from build123d import *

# Parameters (mm, degrees)
SKETCH1_W               = 50.8
SKETCH1_H               = 36.83
BOSS_EXTRUDE1_DEPTH     = 8.89
SKETCH2_W               = 36.83
SKETCH2_H               = 8.89
BOSS_EXTRUDE2_DEPTH     = 0.254
SKETCH3_W               = 4.318
SKETCH3_H               = 10.16
BOSS_EXTRUDE3_DEPTH     = 20.32
CUT_EXTRUDE1_DEPTH      = 54.86357322
CUT_EXTRUDE1_DEPTH_BACK = 54.86357322
SKETCH4_R               = 2.54
FILLET1_R               = 3.81
SKETCH18_5_W            = 20.32
SKETCH18_5_H            = 2.54
CUT_EXTRUDE2_DEPTH      = 51.556369539
SKETCH7_W               = 20.32
SKETCH7_H               = 2.54
CUT_EXTRUDE3_DEPTH      = 51.556369539
SKETCH18_16_R           = 1.27
BOSS_EXTRUDE4_DEPTH     = 6.35
FILLET2_R               = 2.032


with BuildPart() as part:
    # Sketch1 → Boss-Extrude1 (new body)
    with BuildSketch(Plane(origin=(0, 0, 0), x_dir=(1, 0, 0), z_dir=(0, 1, 0))):
        Rectangle(SKETCH1_W, SKETCH1_H)
    extrude(amount=-BOSS_EXTRUDE1_DEPTH)

    # Sketch2 → Boss-Extrude2 (add)
    with BuildSketch(Plane(origin=(25.4, 0, 0), x_dir=(0, 0, -1), z_dir=(1, 0, 0))):
        with Locations((0, -4.445)):
            Rectangle(SKETCH2_W, SKETCH2_H)
    extrude(amount=BOSS_EXTRUDE2_DEPTH)

    # Sketch3 → Boss-Extrude3 (add)
    with BuildSketch(Plane(origin=(25.654, 0, 0), x_dir=(0, 0, -1), z_dir=(1, 0, 0))):
        with Locations((-5.588, -5.08)):
            Rectangle(SKETCH3_W, SKETCH3_H)
        with Locations((5.588, -5.08)):
            Rectangle(SKETCH3_W, SKETCH3_H)
    extrude(amount=BOSS_EXTRUDE3_DEPTH)

    # Sketch4 → Cut-Extrude1 (cut, two sides: drawn at the far end of the back side and taken through both)
    with BuildSketch(Plane(origin=(0, 0, -7.747), x_dir=(-1, 0, 0), z_dir=(0, 0, -1)).offset(-CUT_EXTRUDE1_DEPTH_BACK)):
        with Locations((-40.894, -4.445)):
            Circle(SKETCH4_R)
    extrude(amount=CUT_EXTRUDE1_DEPTH + CUT_EXTRUDE1_DEPTH_BACK, mode=Mode.SUBTRACT)

    # Fillet1
    fillet1_edges = [part.edges().sort_by_distance(p)[0] for p in [
        (45.974, 0, 5.588),
        (45.974, -10.16, 5.588),
        (45.974, 0, -5.588),
        (45.974, -10.16, -5.588),
    ]]
    fillet(fillet1_edges, radius=FILLET1_R)

    # Sketch18_5 → Cut-Extrude2 (cut, through all)
    with BuildSketch(Plane(origin=(0, 0, 0), x_dir=(1, 0, 0), z_dir=(0, 1, 0))):
        with Locations((12.7, 16.256)):
            Rectangle(SKETCH18_5_W, SKETCH18_5_H)
    extrude(amount=-CUT_EXTRUDE2_DEPTH, mode=Mode.SUBTRACT)

    # Sketch7 → Cut-Extrude3 (cut, through all)
    with BuildSketch(Plane(origin=(0, 0, 0), x_dir=(1, 0, 0), z_dir=(0, 1, 0))):
        with Locations((12.7, -16.256)):
            Rectangle(SKETCH7_W, SKETCH7_H)
    extrude(amount=-CUT_EXTRUDE3_DEPTH, mode=Mode.SUBTRACT)

    # Sketch18_16 → Boss-Extrude4 (add)
    with BuildSketch(Plane(origin=(0, 0, 0), x_dir=(1, 0, 0), z_dir=(0, 1, 0))):
        with Locations(Location((-19.304, -14.732, 0), (0, 0, 270))):
            Circle(SKETCH18_16_R)
        with Locations(Location((-19.304, 14.732, 0), (0, 0, 270))):
            Circle(SKETCH18_16_R)
    extrude(amount=BOSS_EXTRUDE4_DEPTH)

    # Fillet2
    fillet2_edges = [part.edges().sort_by_distance(p)[0] for p in [
        (-19.304, 0, 13.462),
        (-19.304, 0, -16.002),
    ]]
    fillet(fillet2_edges, radius=FILLET2_R)


solid = part.part
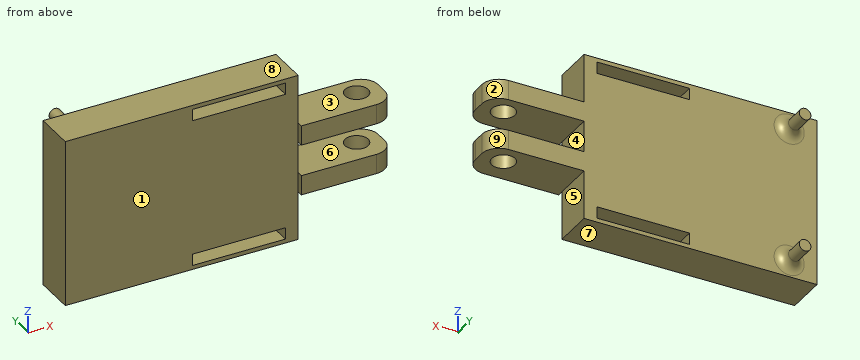
Could you check a few things on this model? Use its own coordinates, in mm. Face numbers are marked on the shaded views. A direction names the side the tool comes from. Give positions to 0.01 mm unless a question says otherwise; leave off trailing zeros. Write each loop counter-clockwise with the first axis right and the second up, starting at its lowest first coordinate (ties: lowest second). Pieces come first, ordered by that corner, then holes. Notation, with made-up numbers: (56.5, 53) -> (98.5, 53) arc R24 ccw to (98.5, 79) -> close; hole circle Ø6 at (39, 84.5). An arc over 180 degrees is marked (long way). Answer as a JSON object with one key per item and string values.
Q1. Which directions (+Z, -Z, +X, -X, +Y, -Y) give clear straight access to the entire face, cutting with the end or side of a thin tool? Please do the marked faces 1, 2, 3, 4 and 5.
Taken from the geometry:
{"face 1": "+Z, -Z, -X, -Y", "face 2": "+Z, -Z, +X, +Y", "face 3": "+Z, +X, +Y, -Y", "face 4": "+X, +Y, -Y", "face 5": "-Z, +X, +Y, -Y"}
Q2. Suppose I cut it at C-C on z = 5. Write out the boundary of the cut face in (x, y) (3 decimals).
Taken from the geometry:
{"outline": "(-25.4, -8.89) -> (25.654, -8.89) -> (25.654, -10.16) -> (42.164, -10.16) arc R3.81 ccw to (45.974, -6.35) -> (45.974, -3.81) arc R3.81 ccw to (42.164, 0) -> (-25.4, 0) -> close; hole circle Ø5.08 at (40.894, -4.445)"}
Q3. Suppose I cut it at A-A on x = 27.5. Write out the boundary of the cut face in (y, z).
Taken from the geometry:
{"outline": "(-10.16, -7.75) -> (0, -7.75) -> (0, -3.43) -> (-10.16, -3.43) -> close; (-10.16, 3.43) -> (0, 3.43) -> (0, 7.75) -> (-10.16, 7.75) -> close"}
Q4. Will these pins go through, and if not, where does the flat tip stop? pin 1 Ø0.6 at (y, z) = (-9.5, 5.5) entering from -X; pin 2 Ø3 at (y, z) = (-4, -17) entering from +X; pin 3 Ø6 at (x, z) = (-13.5, 0) entering from +Y.
Taken from the geometry:
{"pin 1": "stops at x = 25.65", "pin 2": "stops at x = 25.65", "pin 3": "stops at y = 0"}
Q5. We'd pull the mould along Z, two halves only. Please class the marked faces 6, 7, 8 and 9: released by +Z, released by -Z, zero draft, split by the parting line, or undercut.
Taken from the geometry:
{"face 6": "undercut", "face 7": "released by -Z", "face 8": "released by +Z", "face 9": "zero draft"}
Q6. Suppose I cut it at B-B on x = 13. Write out the boundary of the cut face in (y, z) (3 decimals).
Taken from the geometry:
{"outline": "(-8.89, -18.415) -> (0, -18.415) -> (0, -17.526) -> (-8.89, -17.526) -> close; (-8.89, -14.986) -> (0, -14.986) -> (0, 14.986) -> (-8.89, 14.986) -> close; (-8.89, 17.526) -> (0, 17.526) -> (0, 18.415) -> (-8.89, 18.415) -> close"}
Q7. Please list where these lines run through material, in increasing order: L1, parallel to Z at x = 3, y = -6 (3 decimals); L2, parallel to X at y = -6, z = 16; L3, parallel to Z at x = 43, y = -8.
Taken from the geometry:
{"L1": "z = -18.415 to -17.526, -14.986 to 14.986, 17.526 to 18.415", "L2": "x = -25.4 to 2.54, 22.86 to 25.65", "L3": "z = -7.75 to -3.43, 3.43 to 7.75"}
Q8. Suppose I cut it at D-D on y = -3. Write out the boundary of the cut face in (x, z) (3 decimals), then the cut area to 3 significant figures.
Taken from the geometry:
{"outline": "(-25.4, -18.415) -> (25.654, -18.415) -> (25.654, -7.747) -> (38.805, -7.747) -> (38.805, -3.429) -> (25.654, -3.429) -> (25.654, 3.429) -> (38.805, 3.429) -> (38.805, 7.747) -> (25.654, 7.747) -> (25.654, 18.415) -> (-25.4, 18.415) -> close; (42.983, -7.747) -> (45.887, -7.747) -> (45.887, -3.429) -> (42.983, -3.429) -> close; (42.983, 3.429) -> (45.887, 3.429) -> (45.887, 7.747) -> (42.983, 7.747) -> close; hole (2.54, -17.526) -> (22.86, -17.526) -> (22.86, -14.986) -> (2.54, -14.986) -> close; hole (2.54, 14.986) -> (22.86, 14.986) -> (22.86, 17.526) -> (2.54, 17.526) -> close", "area": "1,920 mm²"}
